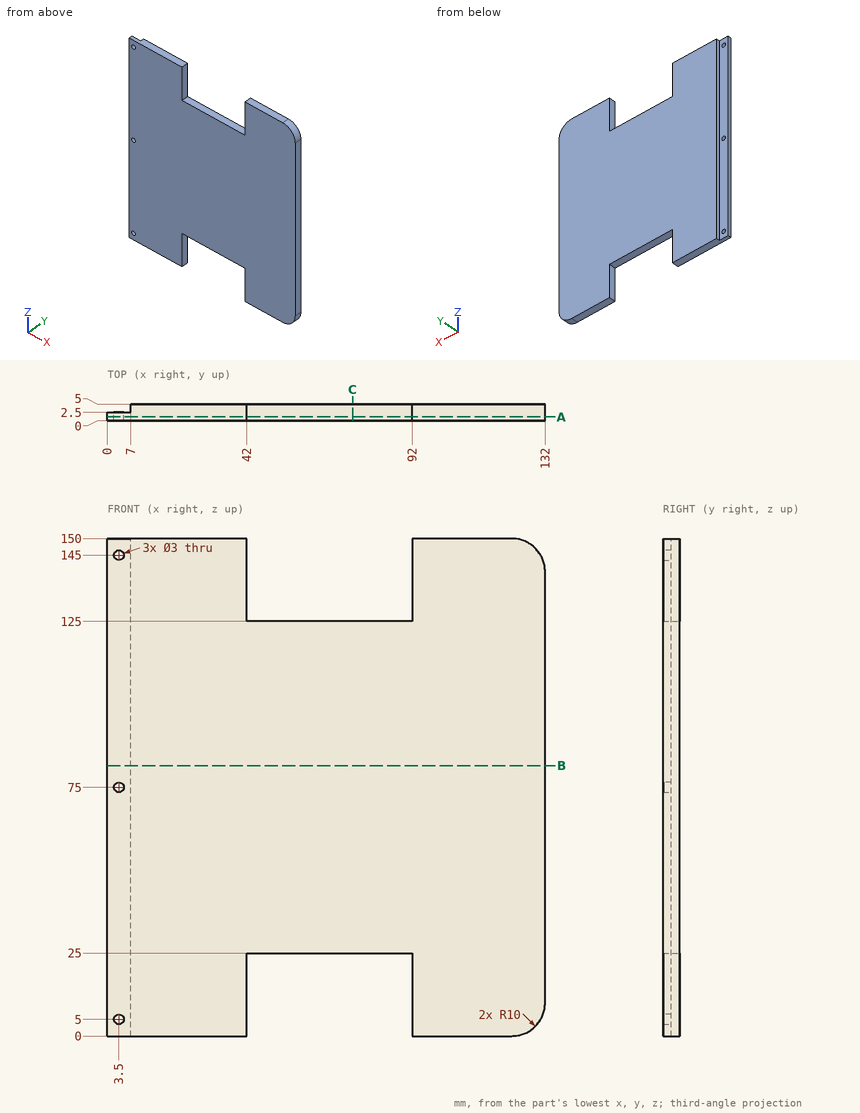
Check sheet for the drawn part. Datum: minimum x, y, z corner. Units: mm. Round coordinates to 2 decimals unless told otherwise and drop trailing zeros. Order: outer loops, then holes, each group sorted by start corner. A loop starts at its lowest first (then second) coordinate and runs counter-clockwise, first axis right, second up. Notation, with made-up numbers: M 21.5,89 L 70.5,89 A5 cw 70.5,93 Z; hole C 72,17 d2. An arc over 180 degrees is marked long. Write each question's results on one line, items separated by ' | '. Start each with the question number.
1. Cross-section at A-A on y = 1.15. Record the boundary of the cut face in (x, z).
2. Material ranges on L1, parallel to X at y = 0.6, z = 135.5; L2, parallel to X at y = 3.2, z = 12; L3, parallel to X at y = 4.85, z = 77, recorded low to high. Write a range as from..to.
3. Cross-section at C-C on x = 74. Record the boundary of the cut face in (y, z), plus the area to 3 significant figures.
4. Go/stop test with flat-tipped pins: P1, Ø5, axis at x = 3.5, z = 5, coming from the +Y side; P2, Ø2.5, axis at x = 3.5, z = 75, coming from the -Y side; P3, Ø2.5, axis at x = 77, y = 3.5, coming from the -Z side; P4, Ø0.8, axis at y = 3.5, z = 42, coming from the -X side. Record where each tip stops, or that it passes through.
5. Cross-section at B-B on z = 81.5. Record the boundary of the cut face in (x, y), plus the area to 4 significant figures.
Resolved:
1) outline: M 0,0 L 42,0 L 42,25 L 92,25 L 92,0 L 122,0 A10 ccw 132,10 L 132,140 A10 ccw 122,150 L 92,150 L 92,125 L 42,125 L 42,150 L 0,150 Z; hole C 3.5,5 d3; hole C 3.5,75 d3; hole C 3.5,145 d3
2) L1: 0..42, 92..132 | L2: 7..42, 92..132 | L3: 7..132
3) outline: M 0,25 L 5,25 L 5,125 L 0,125 Z | area: 500 mm2
4) P1: y = 2.5 | P2: through | P3: z = 25 | P4: x = 7
5) outline: M 0,0 L 132,0 L 132,5 L 7,5 L 7,2.5 L 0,2.5 Z | area: 642.5 mm2
